Read the model definition and answer for the solid it produces. Units are mm, in the model's axes. Face numbers are marked on the shaded views. A direction names the side the tool comes from. Round coordinates to 2 decimals unless told otherwise and drop trailing zeros. Loops run counter-clockwise (first coordinate to the right, second up) from the corner with the lowest first, then second, coordinate; pieces in that order, holes last. Notation, with made-up numbers: (51.5, 33.25) - (55.5, 33.25) arc R16 ccw to (55.5, 46.25) - close; hole circle Ø3 at (-39.5, -31.75). An arc over 180 degrees is marked (long way). Use CSV: the item, a comma, the result in double quotes. Start each with the question number.
1. Find section A-A (z = 41). Give the vertices of the cut face in (x, y).
2. A tool of negligible diameter and unlimited length cuts with its end or side. For the marked faces 5, 6 and 7, from which of +Z, -Z, +X, -X, +Y, -Y can it reach the whole face along a straight path? Write none if from no direction.
3. Consider line 1 along Y through (x, z) = (32, 22.5); line 2 along X through (y, z) = (-16.5, 30); line 3 along Y through (x, z) = (51, 3). Determine where each line is inside the solid, lowest interval first.
4. Determine the mould class of the marked faces 1, 2, 3 and 4 for opening direction Y: +Y half, -Y half, draft (parallel to the pull), parting line (faces both ways), or undercut.
5. Given pin 1 Ø8.5 at (x, y) = (77.5, -4.5) entering from +Z; pin 2 Ø6.5 at (x, y) = (107, -26) entering from -Z; pin 3 Ø2.5 at (x, y) = (82.5, -47.5) entering from -Z, each flat-ended and moving along its own axis, determine where each tip first touches the part or whether it passes through.
6. Find section D-D (z = 55.5). Give the vertices of the cut face in (x, y), and give its area (3 significant figures).
7. Find section B-B (y = -41). Give the vertices of the cut face in (x, z), and give its area (3 significant figures).
8. Find section C-C (x = 75). Give the vertices of the cut face in (y, z).
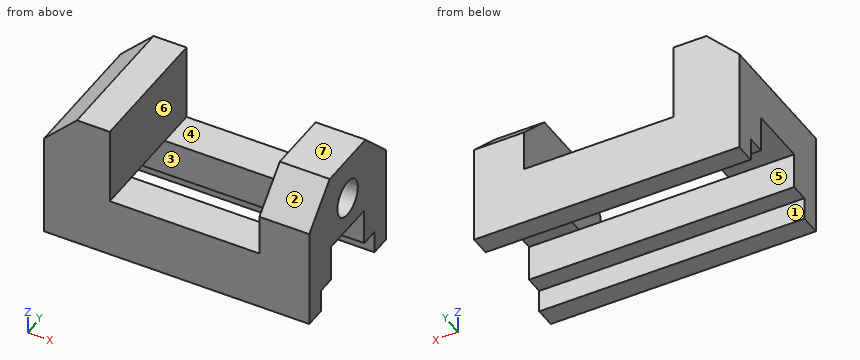
from build123d import *

# Parameters (mm, degrees)
F0_W      = 117
F0_H      = 60
F1_DEPTH  = 60
F2_W      = 66
F2_H      = 34
F3_DEPTH  = 60.001
F5_DEPTH  = 60.001
F7_DEPTH  = 117.001
F9_DEPTH  = 22
F10_R     = 8
F11_DEPTH = 22


with BuildPart() as f1:
    # F0 (on Front) → F1 (new body)
    with BuildSketch(Plane.XZ):
        with Locations((58.5, 30)):
            Rectangle(F0_W, F0_H)
    extrude(amount=F1_DEPTH)

    # F2 (on face) → F3 (cut, through all)
    with BuildSketch(Plane.XZ.offset(60)):
        with Locations((62, 43)):
            Rectangle(F2_W, F2_H)
    extrude(amount=-F3_DEPTH, mode=Mode.SUBTRACT)

    # F4 (on face) → F5 (cut, through all)
    with BuildSketch(Plane.XZ.offset(60)):
        Polygon((0, 45.5), (14.5, 60), (0, 60), align=None)
    extrude(amount=-F5_DEPTH, mode=Mode.SUBTRACT)

    # F6 (on face) → F7 (cut, through all)
    with BuildSketch(Plane.YZ.offset(117)):
        Polygon((-51, 10), (-51, 0), (-9, 0), (-9, 10), (-17, 10), (-17, 26), (-43, 26), (-43, 10), align=None)
    extrude(amount=-F7_DEPTH, mode=Mode.SUBTRACT)

    # F8 (on face) → F9 (cut)
    with BuildSketch(Plane.YZ.offset(117)):
        Polygon((-44, 60), (-60, 60), (-60, 44), align=None)
        Polygon((0, 60), (-16, 60), (0, 44), align=None)
    extrude(amount=-F9_DEPTH, mode=Mode.SUBTRACT)

    # F10 (on face) → F11 (cut)
    with BuildSketch(Plane.YZ.offset(117)):
        with Locations((-30, 41)):
            Circle(F10_R)
    extrude(amount=-F11_DEPTH, mode=Mode.SUBTRACT)


solid = f1.part
Filled sheet:
1,outline,"(0, -60) - (29, -60) - (29, 0) - (0, 0) - close; (95, -60) - (117, -60) - (117, -38) - (95, -38) - close; (95, -22) - (117, -22) - (117, 0) - (95, 0) - close"
2,face 5,"-Z, +X, -X"
2,face 6,"+Z, +Y, -Y"
2,face 7,"+Z, +X, -X, +Y, -Y"
3,line 1,"y = -60 to -43, -17 to 0"
3,line 2,"x = 0 to 29, 95 to 117"
3,line 3,"y = -60 to -51, -9 to 0"
4,face 1,"undercut"
4,face 2,"-Y half"
4,face 3,"undercut"
4,face 4,"draft"
5,pin 1,"stops at z = 26"
5,pin 2,"stops at z = 26"
5,pin 3,"stops at z = 10"
6,outline,"(10, -60) - (29, -60) - (29, 0) - (10, 0) - close; (95, -48.5) - (117, -48.5) - (117, -11.5) - (95, -11.5) - close"
6,area,"1,950 mm²"
7,outline,"(0, 26) - (29, 26) - (29, 60) - (14.5, 60) - (0, 45.5) - close; (95, 26) - (117, 26) - (117, 60) - (95, 60) - close"
7,area,"1,630 mm²"
8,outline,"(-60, 0) - (-51, 0) - (-51, 10) - (-43, 10) - (-43, 26) - (-60, 26) - close; (-17, 10) - (-9, 10) - (-9, 0) - (0, 0) - (0, 26) - (-17, 26) - close"
